Model file for the job. Use its own axes, mm. Face numbers are marked on the shaded views. A direction names the side the tool comes from. Round coordinates to 2 decimals unless told otherwise and drop trailing zeros. Order: outer loops, then holes, each group sorted by start corner. A loop starts at its lowest first (then second) coordinate and runs counter-clockwise, first axis right, second up. Notation, with made-up numbers: (-4, -6) - (12, -6) arc R12 cw to (12, 13) - close; hole circle Ø11 at (11, -38). An arc over 180 degrees is marked (long way). Put each result on its own line as item: value. Start each with the question number.
Item 1: Saw through at B-B on y = 0. List the corners of the cut face in (x, z) (3 decimals).
Item 2: Probe probe 1 along Z at (x, y) = (28, 7.5) (3 decimals); probe 2 along Y at (x, z) = (-10, -26.5); probe 3 along X at (y, z) = (16.5, -24.5). List the from-to ranges inside material, lowest first.
Item 3: Pin check, flat tips, straight feed: pin 1 Ø8 at (y, z) = (8, -17.5) entering from -X; pin 2 Ø5 at (x, z) = (10.5, -13.5) entering from +Y; pin 3 Ø8 at (y, z) = (12.5, -12.5) entering from +X; pin 4 Ø4 at (y, z) = (33.5, -12) entering from -X. Stop position of each tip, or through.
Item 4: Which spindle directions (+Z, -Z, +X, -X, +Y, -Y) get a long thin tool onto all of the face, cutting with end or side? Do the marked faces 1 and 2. Say none if no direction does.
Item 5: Saw through at C-C on z = -22. List the corners of the cut face in (x, y), plus the area to 3 significant figures.
Item 6: Saw through at D-D on z = -11. List the corners of the cut face in (x, y), plus the area to 3 significant figures.
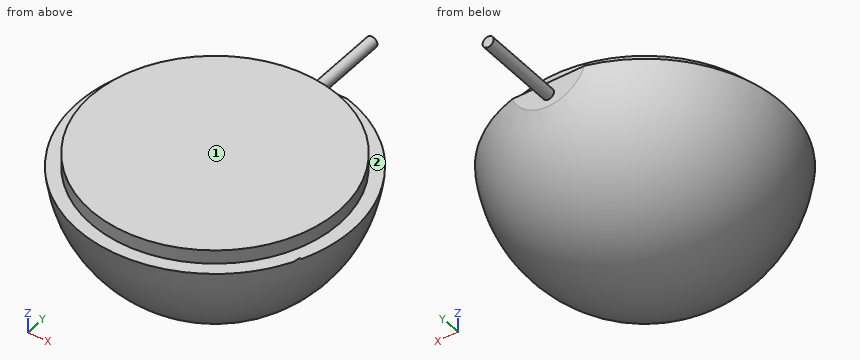
Autodesk Inventor part; units mm, degrees
ref_plane "YZ Plane" through (0, 0, 0) normal (1, 0, 0) x (0, 1, 0)
ref_plane "XZ Plane" through (0, 0, 0) normal (0, 1, 0) x (-1, 0, 0)
ref_plane "XY Plane" through (0, 0, 0) normal (0, 0, 1) x (1, 0, 0)
sketch "Sketch6" plane through (0, 0, 0) normal (0, 0, 1) x (1, 0, 0)
  arc A0 (-31.75, 0) -> (31.75, 0) centre (0, 0) ccw
  line L0 (-31.75, 0) -> (31.75, 0)
revolve "Revolution2" add sketch "Sketch6" angle 180 about axis through (-31.75, 0, 0) along (1, 0, 0)
sketch "Sketch9" plane through (0, 0, 0) normal (0, 0, 1) x (1, 0, 0)
  circle A0 centre (0, 0) radius 31.75
extrude "Extrusion5" cut sketch "Sketch9" against normal blind 3.175
sketch "Sketch10" plane through (0, 0, -3.175) normal (0, 0, 1) x (1, 0, 0)
  circle A0 centre (0, 0) radius 28.575
extrude "Extrusion6" add sketch "Sketch10" along normal blind 3.175
sketch "Sketch11" plane through (0, 0, 0) normal (0, 1, 0) x (-1, 0, 0)
  arc A0 (-31.7973, 0) -> (31.7973, 0) centre (0, 0) ccw
  line L0 (31.7973, 0) -> (-31.7973, 0)
  line L1 (-31.5909, -3.175) -> (31.5909, -3.175)
extrude "Extrusion7" cut sketch "Sketch11" along normal blind 30.48 and the other way blind 31.75 keep common part
sketch "Sketch12" plane through (0, 30.48, 0) normal (0, 1, 0) x (1, 0, 0)
  line L0 (28.575, 3.175) -> (-28.575, 3.175)
  line L1 (0, 3.175) -> (0, 8.89)
  arc A0 (8.3037, 3.175) -> (-8.3037, 3.175) centre (0, 0) ccw
  line L2 (0, 3.175) -> (0, 6.0325)
  circle A1 centre (0, 6.0325) radius 1.27
  dimension "d29" = 5.715
  dimension "d30" = 2.8575
  dimension "d31" = 2.54
extrude "Extrusion8" add sketch "Sketch12" along normal blind 19.05 contours A1 L1 | L1 A1
properties part number "bulb turning point"
Results found:
1. outline: (-31.591, -3.175) arc R31.75 ccw to (31.591, -3.175) - (28.575, -3.175) - (28.575, 0) - (-28.575, 0) - (-28.575, -3.175) - close
2. probe 1: z = -12.954 to -3.175
2. probe 2: y = -14.35 to 14.35
2. probe 3: x = -11.64 to 11.64
3. pin 1: stops at x = -27.85
3. pin 2: stops at y = 28.19
3. pin 3: stops at x = 28.65
3. pin 4: passes through
4. face 1: +Z, +X, -X, +Y, -Y
4. face 2: +Z
5. outline: circle Ø45.78 at (0, 0)
5. area: 1,650 mm²
6. outline: circle Ø59.57 at (0, 0)
6. area: 2,790 mm²
